Input: part model. Units: mm. Frame: model coordinates. A direction names the side the tool comes from. Give positions to 0.01 mm unless a question says otherwise; leave off trailing zeros. Loops run counter-clockwise (first coordinate to the right, second up) from the corner with the lowest first, then second, coordinate; pieces in that order, holes last. Notation, with made-up numbers: M 65,32.5 L 110,32.5 A9 cw 110,41.5 Z; hole C -11.75,1 d1. An arc over 180 degrees is marked long. Return JSON: item names as keys, results as strings. Group by question number.
Autodesk Fusion 360 part; units mm, degrees
sketch "Sketch1" plane through (0, 0, 0) normal (0, 0, 1) x (1, 0, 0)
  circle A0 centre (5, 5) radius 4.75
  dimension "d1" = 9.5
extrude "Extrude1" add sketch "Sketch1" along normal blind 20
sketch "Sketch2" plane through (0, 0, 20) normal (0, 0, 1) x (-1, 0, 0)
  circle A0 centre (-5, -5) radius 4.75
  circle A1 centre (-5, -5) radius 2.875
  dimension "d4" = 5.75
extrude "Extrude2" cut sketch "Sketch2" against normal blind 3.15 contours A1
sketch "Sketch3" plane through (0, 0, 16.85) normal (0, 0, 1) x (-1, 0, 0)
  circle A0 centre (-5, -5) radius 2.875
  circle A1 centre (-5, -5) radius 1.6
  dimension "d7" = 3.2
extrude "Extrude3" cut sketch "Sketch3" against normal blind 0.85 contours A1
sketch "Sketch4" plane through (0, 0, 0) normal (0, 0, -1) x (1, 0, 0)
  circle A0 centre (5, -5) radius 4.75
  circle A1 centre (5, -5) radius 1.625
  dimension "d10" = 3.25
extrude "Extrude4" cut sketch "Sketch4" against normal blind 3 contours A1
sketch "Sketch6" plane through (0, 0, 3) normal (0, 0, -1) x (1, 0, 0)
  circle A0 centre (5, -5) radius 1.625
  circle A1 centre (4.5, -4.5) radius 0.65
  circle A2 centre (5.5, -5.5) radius 0.65
  dimension "d13" = 1.3
  dimension "d14" = 1.3
sketch "Sketch7" plane through (0, 0, 0) normal (0, 0, -1) x (1, 0, 0)
  circle A0 centre (5, -5) radius 1.625
  circle A1 centre (5, -5) radius 4.75
extrude "Extrude5" add sketch "Sketch6" along normal blind 20 contours A1
extrude "Extrude6" add sketch "Sketch6" along normal blind 20 contours A2
Item 1: Section D-D, the plane z = 6. Return loops of the section in (x, y).
Item 2: Pull-direction query (X, two-part tool) for faces 4 (the face through (3.802, 3.902, 1.479)), 5 (the face through (7.554, 0.995, 9.86)), 6 (the face through (5.5, 5.5, -17)); classes: pulls with the +X half, pulls with the -X half, needs draft (parallel to the pull), parting line crosses it, or undercut.
Item 3: Material intervals for line 1 (Y direction, x = 5, z = 2.05) (3 decimals); line 2 (Y direction, x = 5, z = 16.4); line 3 (Y direction, x = 5, z = 17.55) (3 decimals), sorted ascending. Write a range as from..to.
Item 4: Section B-B, the plane x = 4.25. Return loops of the section in (y, z), then the cut area to 3 significant figures.
Item 5: Section C-C, the plane y = 4.5. Return loops of the section in (x, z).
Item 6: Reachability of faces 1 (the face through (3.76, 6.24, 16.85)), 2 (the face through (4.5, 4.5, -17)), 3 (the face through (7, 5, 0)) from +Z, -Z, +X, -X, +Y, -Y: full face, straight path, thin tool, end or side. Return the list, or none.
Item 7: First-contact query: pin 1 Ø1 at (x, z) = (4, 14) entering from -Y; pin 2 Ø1.5 at (x, y) = (7.5, 4) entering from -Z; pin 3 Ø1.9 at (x, y) = (5, 5) entering from +Z; pin 4 Ø1 at (y, z) = (8.5, -9.5) entering from -X. Flat tips, straight axial feed; report the tip coordinate or a pass-through.
Item 8: Section A-A, the plane z = -12. Return loops of the section in (x, y).
Answer below:
{
 "1": {"outline": "C 5,5 d9.5"},
 "2": {"face 4": "undercut", "face 5": "parting line crosses it", "face 6": "needs draft"},
 "3": {"line 1": "0.25..3.375, 4.085..4.915, 5.085..5.915, 6.625..9.75", "line 2": "0.25..3.4, 6.6..9.75", "line 3": "0.25..2.125, 7.875..9.75"},
 "4": {"outline": "M 0.31,0 L 3.56,0 L 3.56,3 L 3.9,3 L 3.9,-17 L 5.1,-17 L 5.1,3 L 6.44,3 L 6.44,0 L 9.69,0 L 9.69,20 L 7.78,20 L 7.78,16.85 L 6.41,16.85 L 6.41,16 L 3.59,16 L 3.59,16.85 L 2.22,16.85 L 2.22,20 L 0.31,20 Z", "area": "183 mm^2"},
 "5": {"outline": "M 0.28,0 L 3.45,0 L 3.45,3 L 3.85,3 L 3.85,-17 L 5.15,-17 L 5.15,3 L 6.55,3 L 6.55,0 L 9.72,0 L 9.72,20 L 7.83,20 L 7.83,16.85 L 6.52,16.85 L 6.52,16 L 3.48,16 L 3.48,16.85 L 2.17,16.85 L 2.17,20 L 0.28,20 Z"},
 "6": {"face 1": "+Z", "face 2": "-Z, +X, -X, +Y, -Y", "face 3": "-Z"},
 "7": {"pin 1": "y = 0.28", "pin 2": "z = 0", "pin 3": "z = 16", "pin 4": "through"},
 "8": {"outline": "C 4.5,4.5 d1.3; C 5.5,5.5 d1.3"}
}
